Part print with two shaded views. Sizes in mm from the minimum x, y, z corner. Round coordinates to 2 decimals unless told otherwise and drop trailing zeros. Loops run counter-clockwise (first coordinate to the right, second up) from the corner with the lowest first, then second, coordinate; pieces in that order, holes last.
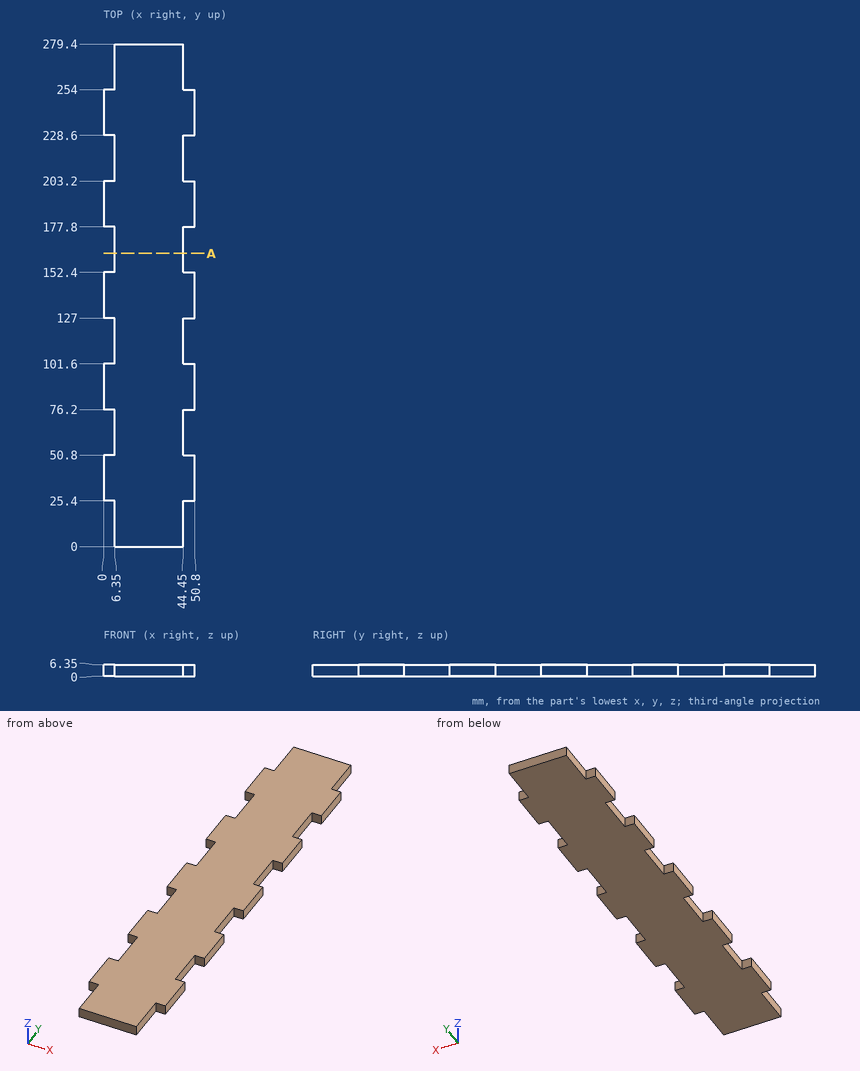
Item 1: Flat gauge pins, fed straight in: P1, Ø3, axis at x = 47.5, z = 2, coming from the -Y side; P2, Ø3, axis at x = 48.5, z = 3, coming from the +Y side; P3, Ø3, axis at y = 66, z = 3, coming from the -X side. Where does each tip first touch, or does it go through?
Verdict:
P1: stops at y = 25.4
P2: stops at y = 254
P3: stops at x = 6.35
Item 2: Wall check: L1, parallel to X at y = 162.5, z = 5. Give the ranges that are in metal, low to high.
Verdict:
L1: x = 6.35 to 44.45
Item 3: Cut at A-A (y = 163). List the corners of the cut face in (x, z).
Verdict:
outline: (6.35, 0) - (44.45, 0) - (44.45, 6.35) - (6.35, 6.35) - close
